```python
from build123d import *

# Parameters (mm, degrees)
SKETCH_1_W          = 160
SKETCH_1_H          = 80
EXTRUDE_1_DEPTH     = 20
HOLE_WIZARD_M10_1_D = 11
MM_1_D              = 10


with BuildPart() as part:
    # 草图1 → 凸台-拉伸1 (new body)
    with BuildSketch(Plane.XY):
        Rectangle(SKETCH_1_W, SKETCH_1_H)
    extrude(amount=EXTRUDE_1_DEPTH)

    # M10 间隙孔1 (through all)
    with Locations(Plane.XY.offset(20)):
        with Locations((-25, 25), (25, -20)):
            Hole(HOLE_WIZARD_M10_1_D / 2)

    # 大小mm 暗销孔1 (through all)
    with Locations(Plane.XY.offset(20)):
        with Locations((25, 25), (-25, -20)):
            Hole(MM_1_D / 2)


solid = part.part
```
Geometry check sheet. Reference: the model listing, model coordinates, mm. Give positions to 0.01 mm unless a question says otherwise; leave off trailing zeros. Order: outer loops, then holes, each group sorted by start corner. A loop starts at its lowest first (then second) coordinate and runs counter-clockwise, first axis right, second up. Notation, with made-up numbers: (15.5, 78) - (70.5, 78) arc R36 ccw to (70.5, 113) - close; hole circle Ø7 at (16.25, -14). An arc over 180 degrees is marked (long way). Write item = value, one per line. Start each with the question number.
1) Gauge pin test, flat end, axial feed: pin 1 Ø6 at (x, y) = (-25, -20) entering from -Z. Record the tip position at first contact, or that the pin passes through.
2) Scan lines: L1, parallel to Y at x = 25, z = 6.75; L2, parallel to Y at x = -25, z = 14.5; L3, parallel to X at y = -21, z = 5.25. Record each from-to range of solid material in increasing order.
3) Draft check along X on faces 1 (the flat face through (-80, -1, 10)), 2 (the cylindrical face through (-21, -23, 10)), 3 (the flat face through (-1, 1, 20)). Enter one of: released by +X, released by -X, zero draft, split by the parting line, or undercut.
4) Section check C-C (z = 2). Enter the section's corners in (x, y).
5) Section check B-B (y = -20). Enter the section's corners in (x, z), then the cut area to 3 significant figures.
6) Section check A-A (x = -25). Enter the section's corners in (y, z).
Geometry check:
q1.pin_1 = through
q2.L1 = -40 to -25.5, -14.5 to 20, 30 to 40
q2.L2 = -40 to -25, -15 to 19.5, 30.5 to 40
q2.L3 = -80 to -29.9, -20.1 to 19.59, 30.41 to 80
q3.face_1 = released by -X
q3.face_2 = undercut
q3.face_3 = zero draft
q4.outline = (-80, -40) - (80, -40) - (80, 40) - (-80, 40) - close; hole circle Ø11 at (-25, 25); hole circle Ø10 at (-25, -20); hole circle Ø11 at (25, -20); hole circle Ø10 at (25, 25)
q5.outline = (-80, 0) - (-30, 0) - (-30, 20) - (-80, 20) - close; (-20, 0) - (19.5, 0) - (19.5, 20) - (-20, 20) - close; (30.5, 0) - (80, 0) - (80, 20) - (30.5, 20) - close
q5.area = 2,780 mm2
q6.outline = (-40, 0) - (-25, 0) - (-25, 20) - (-40, 20) - close; (-15, 0) - (19.5, 0) - (19.5, 20) - (-15, 20) - close; (30.5, 0) - (40, 0) - (40, 20) - (30.5, 20) - close
